```python
from build123d import *

# Parameters (mm, degrees)
F0_W     = 3
F0_H     = 2
F0_W_2   = 1.5
F0_H_2   = 5
F1_DEPTH = 3


with BuildPart() as f1:
    # F0 (on Right) → F1 (new body)
    with BuildSketch(Plane.YZ):
        Polygon((1.5, 5), (1.5, 0), (11.5, 0), (14.5, 0), (14.5, 5), (14.5, 10), (11.5, 10), (1.5, 10), align=None)
        Polygon((17.5, 5), (17.5, 0), (20.5, 0), (30.5, 0), (30.5, 5), (30.5, 10), (20.5, 10), (17.5, 10), align=None)
        with Locations((45, -1)):
            Rectangle(F0_W, F0_H)
        with Locations((0.75, 7.5)):
            Rectangle(F0_W_2, F0_H_2)
        with Locations((-0.75, 7.5)):
            Rectangle(F0_W_2, F0_H_2)
        with Locations((16, 7.5)):
            Rectangle(F0_W, F0_H_2)
        with Locations((32, 7.5)):
            Rectangle(F0_W, F0_H_2)
        with Locations((48, 7.5)):
            Rectangle(F0_W, F0_H_2)
        with Locations((51, -1)):
            Rectangle(F0_W, F0_H)
        with Locations((64, 7.5)):
            Rectangle(F0_W, F0_H_2)
        with Locations((77, -1)):
            Rectangle(F0_W, F0_H)
        with Locations((80, 7.5)):
            Rectangle(F0_W, F0_H_2)
        with Locations((83, -1)):
            Rectangle(F0_W, F0_H)
        with Locations((95.25, 7.5)):
            Rectangle(F0_W_2, F0_H_2)
        with Locations((96.75, 7.5)):
            Rectangle(F0_W_2, F0_H_2)
        with Locations((109, -1)):
            Rectangle(F0_W, F0_H)
        with Locations((112, 7.5)):
            Rectangle(F0_W, F0_H_2)
        with Locations((115, -1)):
            Rectangle(F0_W, F0_H)
        with Locations((128, 7.5)):
            Rectangle(F0_W, F0_H_2)
        with Locations((141, -1)):
            Rectangle(F0_W, F0_H)
        with Locations((144, 7.5)):
            Rectangle(F0_W, F0_H_2)
        with Locations((147, -1)):
            Rectangle(F0_W, F0_H)
        with Locations((160, 7.5)):
            Rectangle(F0_W, F0_H_2)
        with Locations((173, -1)):
            Rectangle(F0_W, F0_H)
        with Locations((176, 7.5)):
            Rectangle(F0_W, F0_H_2)
        with Locations((179, -1)):
            Rectangle(F0_W, F0_H)
        with Locations((191.25, 7.5)):
            Rectangle(F0_W_2, F0_H_2)
        with Locations((192.75, 7.5)):
            Rectangle(F0_W_2, F0_H_2)
        with Locations((13, -1)):
            Rectangle(F0_W, F0_H)
        with Locations((19, -1)):
            Rectangle(F0_W, F0_H)
        Polygon((33.5, 5), (33.5, 0), (43.5, 0), (46.5, 0), (46.5, 5), (46.5, 10), (33.5, 10), align=None)
        Polygon((49.5, 5), (49.5, 0), (52.5, 0), (62.5, 0), (62.5, 5), (62.5, 10), (49.5, 10), align=None)
        Polygon((78.5, 10), (65.5, 10), (65.5, 5), (65.5, 0), (75.5, 0), (78.5, 0), (78.5, 5), align=None)
        Polygon((94.5, 10), (81.5, 10), (81.5, 5), (81.5, 0), (84.5, 0), (94.5, 0), (94.5, 5), align=None)
        Polygon((110.5, 10), (97.5, 10), (97.5, 5), (97.5, 0), (107.5, 0), (110.5, 0), (110.5, 5), align=None)
        Polygon((126.5, 10), (113.5, 10), (113.5, 5), (113.5, 0), (116.5, 0), (126.5, 0), (126.5, 5), align=None)
        Polygon((142.5, 10), (129.5, 10), (129.5, 5), (129.5, 0), (139.5, 0), (142.5, 0), (142.5, 5), align=None)
        Polygon((158.5, 10), (145.5, 10), (145.5, 5), (145.5, 0), (148.5, 0), (158.5, 0), (158.5, 5), align=None)
        Polygon((171.5, 10), (161.5, 10), (161.5, 5), (161.5, 0), (171.5, 0), (174.5, 0), (174.5, 5), (174.5, 10), align=None)
        Polygon((180.5, 10), (177.5, 10), (177.5, 5), (177.5, 0), (180.5, 0), (190.5, 0), (190.5, 5), (190.5, 10), align=None)
    extrude(amount=F1_DEPTH)


solid = f1.part
```
Verification items for the finished model (mm, model axes). A direction names the side the tool comes from. Round coordinates to 2 decimals unless told otherwise and drop trailing zeros. Write each loop counter-clockwise with the first axis right and the second up, starting at its lowest first coordinate (ties: lowest second). Pieces come first, ordered by that corner, then holes.
1. Access from +Z, -Z, +X, -X, +Y, -Y to the whole of each face (thin tool, end or side, straight path). Record for faces 5 (the flat face through (1, 160, 5)), 6 (the flat face through (1, 6, 0)), 7 (the flat face through (1, 109, -2)).
2. Section check A-A on z = 2.25. State how many separate pieces and enclosed holes the cut face has, plus the area to 3 significant figures.
3. Draft check along Y on faces 1 (the flat face through (1, 1.5, 3)), 2 (the flat face through (1, 134, 0)), 3 (the flat face through (1, 179, -2)), 4 (the flat face through (1, 64, 5)). Enter one of: +Y half, -Y half, draft (parallel to the pull), parting line (faces both ways), or undercut.
4. Gauge pin test, flat ends, axial feed: P1, Ø0.9, axis at x = 2, z = 0.5, coming from the +Y side; P2, Ø1.5, axis at x = 1, y = 7.5, coming from the -Z side; P3, Ø0.6, axis at x = 2, z = -1, coming from the -Y side; P4, Ø6, axis at y = 52, z = 4, coming from the -X side. Record the tip position at first contact, or that the pin passes through.
5. Scan lines: L1, parallel to Z at x = 2.9, y = 150.5; L2, parallel to Z at x = 0.85, y = 97. Record each from-to range of solid material in increasing order.
6. Section check B-B on y = 58.5. Enter the section's corners in (x, z), plus the area to 3 significant figures.
Answer:
1. face 5: -Z, +X, -X
1. face 6: -Z, +X, -X, -Y
1. face 7: -Z, +X, -X, +Y, -Y
2. separate pieces: 12
2. enclosed holes: 0
2. area: 468 mm2
3. face 1: -Y half
3. face 2: undercut
3. face 3: draft
3. face 4: undercut
4. P1: stops at y = 190.5
4. P2: stops at z = 0
4. P3: stops at y = 11.5
4. P4: stops at x = 0
5. L1: z = 0 to 10
5. L2: z = 5 to 10
6. outline: (0, 0) - (3, 0) - (3, 10) - (0, 10) - close
6. area: 30.0 mm2
